Verification items for the finished model (mm, model axes). A direction names the side the tool comes from. Coordinates: 2 decimals unless noted, no trailing zeros. Order: outer loops, then holes, each group sorted by start corner. A loop starts at its lowest first (then second) coordinate and runs counter-clockwise, first axis right, second up. Notation, with made-up numbers: M 25.25,5.25 L 49.25,5.25 A25 cw 49.25,44.25 Z; hole C 35.5,-18.75 d10. An arc over 180 degrees is marked long. Use one line per item in the form item = value. Start each with the question number.
```python
from build123d import *

# Parameters (mm, degrees)
SKETCH1_W               = 60
SKETCH1_H               = 150
SKETCH1_W_2             = 50
SKETCH1_H_2             = 140
BOSS_EXTRUDE1_DEPTH     = 10
SKETCH1_2_W             = 60
SKETCH1_2_H             = 150
SKETCH1_2_W_2           = 50
SKETCH1_2_H_2           = 140
SKETCH1_2_W_3           = 12.5
SKETCH1_2_H_3           = 22.5
BOSS_EXTRUDE2_DEPTH     = 2
SKETCH2_W               = 29
SKETCH2_H               = 12
CUT_EXTRUDE1_DEPTH      = 18.7
SKETCH2_3_R             = 2
BOSS_EXTRUDE3_DEPTH     = 3.7
BOSS_EXTRUDE4_DEPTH     = 10
SKETCH4_W               = 34
SKETCH4_H               = 13
CUT_EXTRUDE2_DEPTH      = 164.406517618
CUT_EXTRUDE2_DEPTH_BACK = 164.406517618
CUT_EXTRUDE3_REACH      = 165.272
SKETCH5_W               = 30
SKETCH5_H               = 5
FILLET1_R               = 3


with BuildPart() as part:
    # Sketch1 → Boss-Extrude1 (new body)
    with BuildSketch(Plane(origin=(0, 0, 0), x_dir=(1, 0, 0), z_dir=(0, 1, 0))):
        with Locations((30, -75)):
            Rectangle(SKETCH1_W, SKETCH1_H)
        with Locations((30, -75)):
            Rectangle(SKETCH1_W_2, SKETCH1_H_2, mode=Mode.SUBTRACT)
    extrude(amount=BOSS_EXTRUDE1_DEPTH)

    # Sketch1<2> → Boss-Extrude2 (add)
    with BuildSketch(Plane(origin=(0, 0, 0), x_dir=(1, 0, 0), z_dir=(0, 1, 0))):
        with Locations((30, -75)):
            Rectangle(SKETCH1_2_W, SKETCH1_2_H)
        with Locations((30, -75)):
            Rectangle(SKETCH1_2_W_2, SKETCH1_2_H_2, mode=Mode.SUBTRACT)
        with Locations((30, -75)):
            Rectangle(SKETCH1_2_W_2, SKETCH1_2_H_2)
        with Locations((30, -34.617801795)):
            Rectangle(SKETCH1_2_W_3, SKETCH1_2_H_3)
    extrude(amount=-BOSS_EXTRUDE2_DEPTH)

    # Sketch2 → Cut-Extrude1 (cut)
    with BuildSketch(Plane.ZY):
        with Locations((126.5, 4)):
            Rectangle(SKETCH2_W, SKETCH2_H)
    cut_extrude1 = extrude(amount=-CUT_EXTRUDE1_DEPTH, mode=Mode.SUBTRACT)

    # Sketch2<3> → Boss-Extrude3 (add)
    with BuildSketch(Plane.ZY):
        with Locations(Location((109, 4, 0), (0, 0, 180))):
            Circle(SKETCH2_3_R)
        with Locations(Location((144, 4, 0), (0, 0, 180))):
            Circle(SKETCH2_3_R)
    boss_extrude3 = extrude(amount=BOSS_EXTRUDE3_DEPTH)

    # Mirror1: Cut-Extrude1, Boss-Extrude3 across plane
    add(cut_extrude1.mirror(Plane.ZY.offset(-30)), mode=Mode.SUBTRACT)
    add(boss_extrude3.mirror(Plane.ZY.offset(-30)))

    # Sketch3 → Boss-Extrude4 (add)
    with BuildSketch(Plane(origin=(0, 0, 0), x_dir=(1, 0, 0), z_dir=(0, 1, 0))):
        Polygon((23.7, -107), (5, -107), (5, -112), (18.7, -112), (18.7, -141), (5, -141), (5, -145), (23.7, -145), align=None)
        Polygon((36.3, -107), (36.3, -145), (55, -145), (55, -141), (41.3, -141), (41.3, -112), (55, -112), (55, -107), align=None)
    extrude(amount=BOSS_EXTRUDE4_DEPTH)

    # Sketch4 → Cut-Extrude2 (cut, two sides)
    with BuildSketch(Plane.XZ.offset(2)) as cut_extrude2_sk:
        with Locations((23.75, 11.5)):
            Rectangle(SKETCH4_W, SKETCH4_H)
    extrude(amount=CUT_EXTRUDE2_DEPTH, mode=Mode.SUBTRACT)
    extrude(cut_extrude2_sk.sketch, amount=-CUT_EXTRUDE2_DEPTH_BACK, mode=Mode.SUBTRACT)

    # Sketch5 → Cut-Extrude3 (cut, up to next)
    with BuildSketch(Plane(origin=(0, 0, 0), x_dir=(-1, 0, 0), z_dir=(0, 0, -1)), mode=Mode.PRIVATE) as cut_extrude3_sk1:
        with Locations((-30, 7.5)):
            Rectangle(SKETCH5_W, SKETCH5_H)
    cut_extrude3_tool1 = extrude(cut_extrude3_sk1.sketch, amount=-CUT_EXTRUDE3_REACH, mode=Mode.PRIVATE) & part.part
    add(cut_extrude3_tool1.solids().sort_by_distance((30, 7.5, 0))[0], mode=Mode.SUBTRACT)

    # Fillet1
    fillet1_edges = [part.edges().sort_by_distance(p)[0] for p in [
        (45, 5, 2.5),
        (15, 5, 2.5),
    ]]
    fillet(fillet1_edges, radius=FILLET1_R)


solid = part.part
```
1. Release check for a two-part mould opening along Z. For faces 1 (the flat face through (46, 5, 107)), 2 (the flat face through (30, 4, 150)), 3 (the flat face through (41, 10, 108)) record: pulls with the +Z half, pulls with the -Z half, needs draft (parallel to the pull), parting line crosses it, or undercut.
2. Tool access check on faces 4 (the cylindrical face through (62, 4, 111)), 5 (the flat face through (30, 5, 2)), 6 (the flat face through (23.7, 5, 126)). Record the directions out of +Z, -Z, +X, -X, +Y, -Y that give a thin tool (end or side, any length) a straight path to the whole face; none if there is none.
3. Material ranges on line 1 along Z through (x, y) = (13.5, 2); line 2 along X through (y, z) = (7, 30.5); line 3 along Z through (x, y) = (6, -1), recorded low to high.
4. Cross-section at A-A on x = 27.5. Enter the section's corners in (y, z).
5. Depth check by flat-ended pin: P1, Ø5, axis at y = 6.5, z = 67, coming from the +X side; P2, Ø1, axis at y = 6, z = 132.5, coming from the +X side; P3, Ø2.5, axis at x = 27.5, z = 3.5, coming from the +Y side. Enter the tip coordinate at first touch or a pass-through.
6. Cross-section at B-B on z = 15. Enter the section's corners in (x, y), and give its area (3 significant figures).
7. Cross-section at C-C on z = 96. Enter the section's corners in (x, y).
Final values:
q1.face_1 = undercut
q1.face_2 = pulls with the +Z half
q1.face_3 = needs draft
q2.face_4 = +X
q2.face_5 = -Z, +Y
q2.face_6 = +Y
q3.line_1 = 0 to 5, 107 to 112, 141 to 150
q3.line_2 = 0 to 5, 55 to 60
q3.line_3 = 0 to 112, 141 to 150
q4.outline = M -2,0 L 5,0 L 5,5 L -2,5 Z; M -2,18 L 0,18 L 0,145 L 10,145 L 10,150 L -2,150 Z
q5.P1 = 60
q5.P2 = 41.3
q5.P3 = 5
q6.outline = M 0,-2 L 6.75,-2 L 6.75,0 L 5,0 L 5,10 L 0,10 Z; M 40.75,-2 L 60,-2 L 60,10 L 55,10 L 55,0 L 40.75,0 Z
q6.area = 152 mm2
q7.outline = M 0,-2 L 60,-2 L 60,10 L 55,10 L 55,0 L 5,0 L 5,10 L 0,10 Z
